Can you work these out from the model? Positions are in its coordinate system, mm. Face numbers are marked on the shaded views. A direction names the side the tool comes from. Coordinates: 2 decimals unless noted, no trailing zeros. Order: outer loops, then holes, each group sorted by start corner. A loop starts at its lowest first (then second) coordinate and runs counter-clockwise, first axis right, second up. Notation, with made-up numbers: (12, -28.5) -> (47, -28.5) arc R18 cw to (47, -11.5) -> close; hole circle Ø7 at (16.25, 18.5). An arc over 180 degrees is marked (long way). Write item = value, one per line. Start each with the question number.
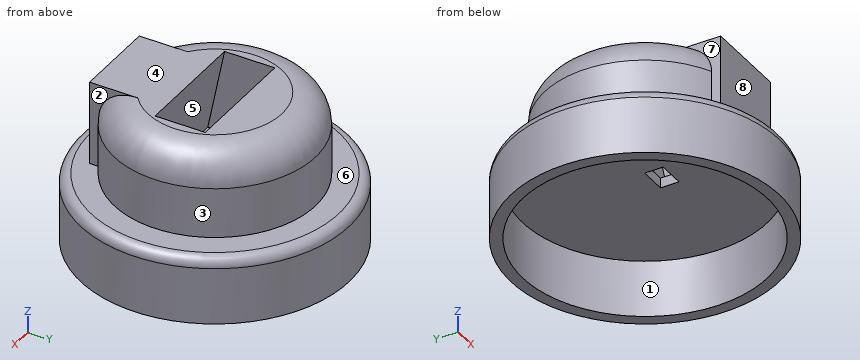
from build123d import *

# Parameters (mm, degrees)
F3_W      = 25
F3_H      = 25
F4_DEPTH  = 25
F5_R      = 10
F6_R      = 3
F7_W      = 35
F7_H      = 15
F8_W      = 35
F8_H      = 15
F10_R     = 36.5
F11_DEPTH = 17
F12_W     = 8
F12_H     = 5.5
F13_DEPTH = 20.001


with BuildPart() as f1:
    # F0 (on Front) → F1 (revolve)
    with BuildSketch(Plane.XZ):
        Polygon((-40, 0), (0, 0), (0, 20), (0, 45), (-30, 45), (-30, 20), (-40, 20), align=None)
    revolve(axis=Axis((0, 0, 32.5), (0, 0, -1)))

    # F3 (on offset) → F4 (join)
    with BuildSketch(Plane.XZ.offset(30)):
        with Locations((0, 32.5)):
            Rectangle(F3_W, F3_H)
    extrude(amount=-F4_DEPTH)

    # F5
    f5_edges = [f1.edges().sort_by_distance(p)[0] for p in [
        (0, 30, 45),
    ]]
    fillet(f5_edges, radius=F5_R)

    # F6
    f6_edges = [f1.edges().sort_by_distance(p)[0] for p in [
        (40, 0, 20),
    ]]
    fillet(f6_edges, radius=F6_R)

    # F7 (on face) → F9 section 0
    with BuildSketch(Plane.XY.offset(45)):
        Rectangle(F7_W, F7_H)
    # F8 (on face) → F9 section 1
    with BuildSketch(Plane.XY.offset(20)):
        with Locations((0, -5)):
            Rectangle(F8_W, F8_H)
    loft(mode=Mode.SUBTRACT)

    # F10 (on face) → F11 (cut)
    with BuildSketch(Plane(origin=(0, 0, 0), x_dir=(1, 0, 0), z_dir=(0, 0, -1))):
        Circle(F10_R)
    extrude(amount=-F11_DEPTH, mode=Mode.SUBTRACT)

    # F12 (on face) → F13 (cut, through all)
    with BuildSketch(Plane.XY.offset(20)):
        with Locations((0, -5)):
            Rectangle(F12_W, F12_H)
    extrude(amount=-F13_DEPTH, mode=Mode.SUBTRACT)


solid = f1.part
(1) Imagine slicing it at B-B (z = 3). Write out the boundary of the cut face in (x, y).
(2) For P1, Ø12.5, axis at x = -6, z = 30, coming from the -Y side; P2, Ø3, axis at x = -31.5, y = 20, coming from the -Z side; P3, Ø0.9, axis at x = -1.5, z = 19, coming from the -Y side; P4, Ø7, axis at y = -20, z = 28, coming from the -X side, each with a flat end and sliding along its axis, tell me the tip position at first contact or that it passes through.
(3) Imagine slicing it at A-A (x = 0). Write out the boundary of the cut face in (y, z).
(4) Imagine slicing it at C-C (z = 19). Write out the boundary of the cut face in (x, y).
(5) For the marked faces 5, 6, 7 and 8, which set-ups out of +Z, -Z, +X, -X, +Y, -Y let a thin tool reach every point of the face, with its end or its side?
(6) If I drill on L1, parallel to X at y = -6.5, z = 17.5; L2, parallel to Z at x = 11, y = 8; L3, parallel to X at y = 1.5, z = 21.5, over which ranges is the centre line in solid material (lowest first)? Write a range as from..to.
(7) Thinking about a two-plate mould opening in X: for the marked faces 1, 2, 3 and 4, which applies, +X half, -X half, draft (parallel to the pull), parting line (faces both ways), or undercut?
Result set:
q1.outline = circle Ø80 at (0, 0); hole circle Ø73 at (0, 0)
q2.P1 = -30
q2.P2 = 0
q2.P3 = -39.54
q2.P4 = -25.05
q3.outline = (-40, 0) -> (-36.5, 0) -> (-36.5, 17) -> (-7.75, 17) -> (-7.75, 20) -> (-12.5, 20) -> (-7.5, 45) -> (-30, 45) -> (-30, 20) -> (-37, 20) arc R3 ccw to (-40, 17) -> close; (-2.25, 17) -> (36.5, 17) -> (36.5, 0) -> (40, 0) -> (40, 17) arc R3 ccw to (37, 20) -> (30, 20) -> (30, 35) arc R10 ccw to (20, 45) -> (7.5, 45) -> (2.5, 20) -> (-2.25, 20) -> close
q4.outline = circle Ø78.47 at (0, 0); hole (-4, -7.75) -> (4, -7.75) -> (4, -2.25) -> (-4, -2.25) -> close
q5.face_5 = none
q5.face_6 = +Z
q5.face_7 = +Z, -X, -Y
q5.face_8 = +Z, +X, -X, -Y
q6.L1 = -39.43..-4, 4..39.43
q6.L2 = 17..45
q6.L3 = -29.96..-17.5, 17.5..29.96
q7.face_1 = undercut
q7.face_2 = +X half
q7.face_3 = parting line
q7.face_4 = draft
